from build123d import *

# Parameters (mm, degrees)
F0_W     = 80
F0_H     = 60
F1_DEPTH = 2
F2_W     = 80
F2_H     = 60
F2_W_2   = 76
F2_H_2   = 56
F3_DEPTH = 20
F4_W     = 13
F4_H     = 12
F4_W_2   = 10
F5_DEPTH = 2


# Not quite as in the source:
# - the program builds the solid bodies; features that only make, move or delete a surface that nothing else refers to are left out


with BuildPart() as f1:
    # F0 (on Top) → F1 (new body)
    with BuildSketch(Plane.XY):
        Rectangle(F0_W, F0_H)
    extrude(amount=F1_DEPTH)

    # F2 (on face) → F3 (join)
    with BuildSketch(Plane.XY.offset(2)):
        Rectangle(F2_W, F2_H)
        Rectangle(F2_W_2, F2_H_2, mode=Mode.SUBTRACT)
    extrude(amount=F3_DEPTH)

    # F4 (on face) → F5 (cut)
    with BuildSketch(Plane.YZ.offset(40)):
        with Locations((-15.5, 13)):
            Rectangle(F4_W, F4_H)
        with Locations((14.4, 13)):
            Rectangle(F4_W_2, F4_H)
    extrude(amount=-F5_DEPTH, mode=Mode.SUBTRACT)


solid = f1.part
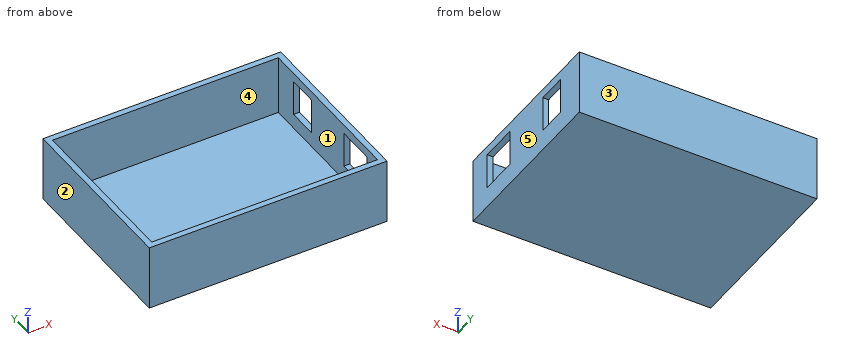
CAD build for the part. Positions are in the model's coordinates, mm. Face numbers are marked on the shaded views. A direction names the side the tool comes from. Round coordinates to 2 decimals unless told otherwise and drop trailing zeros. Loops run counter-clockwise (first coordinate to the right, second up) from the corner with the lowest first, then second, coordinate; pieces in that order, holes last.
(1) Cut at D-D (z = 4.5). Give the cut face in (x, y).
(2) Cut at A-A (z = 8.5). Give the cut face in (x, y), plus the area to 3 significant figures.
(3) Drop a flat-ended pin along its axis: pin 1 (3 mm diameter, centred on x = 16.5, y = 16.5, fed in from +Z). Give the stop position or say it passes through.
(4) Wall check: line 1 along X through (y, z) = (0.5, 17); line 2 along Y through (x, z) = (22, 10); line 3 along Z through (x, y) = (2.5, 24.5). Give the ranges that are in metal, low to high.
(5) Two-plate mould, pull along X, no slides. Class the marked faces 1, 2 and 3: +X half, -X half, draft (parallel to the pull), parting line (faces both ways), or undercut.
(6) Cut at B-B (y = 17.5). Give the cut face in (x, z).
(7) Which spindle directions (+Z, -Z, +X, -X, +Y, -Y) get a long thin tool onto all of the face, cutting with end or side? Do the marked faces 4 and 5. Say none if no direction does.
(8) Cut at C-C (x = -13). Give the cut face in (y, z).
Findings below:
1. outline: (-40, -30) - (40, -30) - (40, 30) - (-40, 30) - close; hole (-38, -28) - (38, -28) - (38, 28) - (-38, 28) - close
2. outline: (-40, -30) - (40, -30) - (40, -22) - (38, -22) - (38, -28) - (-38, -28) - (-38, 28) - (38, 28) - (38, 19.4) - (40, 19.4) - (40, 30) - (-40, 30) - close; (38, -9) - (40, -9) - (40, 9.4) - (38, 9.4) - close
2. area: 498 mm2
3. pin 1: stops at z = 2
4. line 1: x = -40 to -38, 38 to 40
4. line 2: y = -30 to -28, 28 to 30
4. line 3: z = 0 to 2
5. face 1: undercut
5. face 2: -X half
5. face 3: draft
6. outline: (-40, 0) - (40, 0) - (40, 7) - (38, 7) - (38, 2) - (-38, 2) - (-38, 22) - (-40, 22) - close; (38, 19) - (40, 19) - (40, 22) - (38, 22) - close
7. face 4: +Z
7. face 5: +Z, -Z, +X, +Y, -Y
8. outline: (-30, 0) - (30, 0) - (30, 22) - (28, 22) - (28, 2) - (-28, 2) - (-28, 22) - (-30, 22) - close
